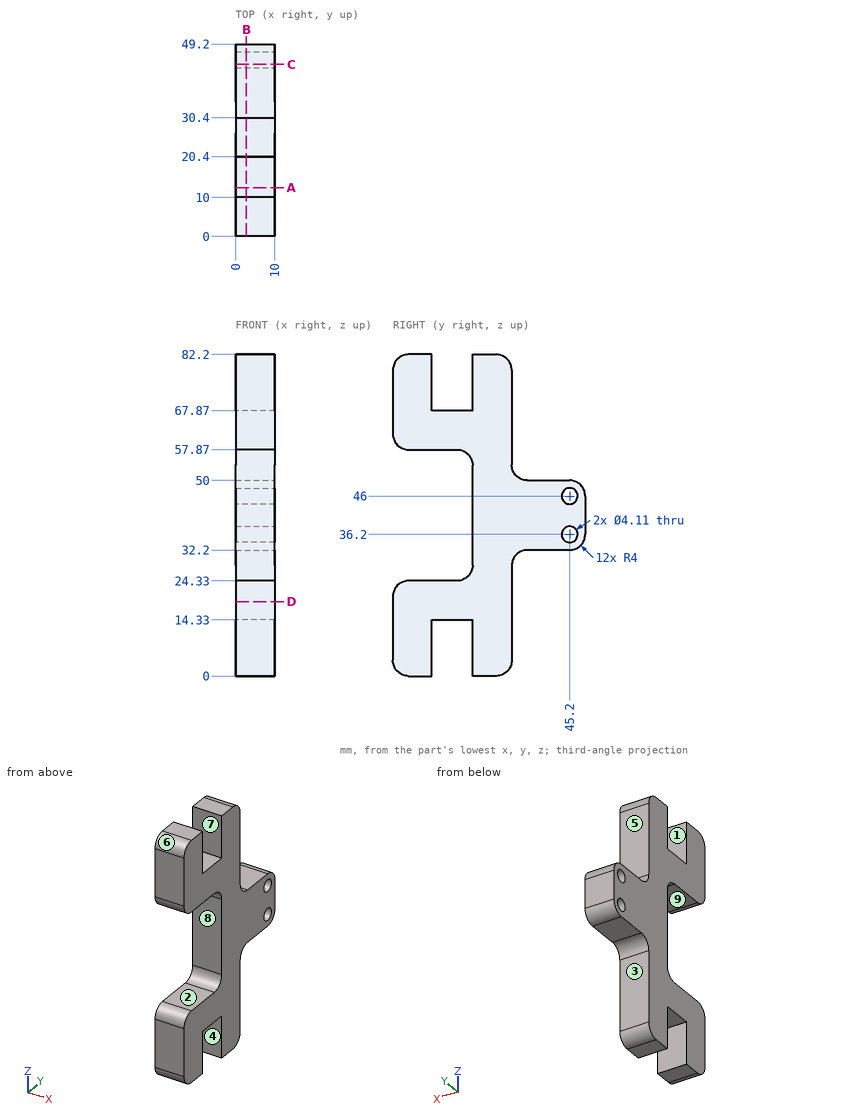
Drawing for the job (mm, zero at the part's lowest x, y, z). A direction names the side the tool comes from. Round coordinates to 2 decimals unless told otherwise and drop trailing zeros. Loops run counter-clockwise (first coordinate to the right, second up) from the corner with the lowest first, then second, coordinate; pieces in that order, holes last. Notation, with made-up numbers: M 45,0.25 L 65,0.25 A11 ccw 65,9.25 Z; hole C -29,63 d10. An arc over 180 degrees is marked long. Use a Markdown table: item, result. Add a question column.
(1) Flat gauge pins, fed straight in: pin 1 (5 mm diameter, centred on x = 4, y = 39, fed in from +Z); pin 2 (6 mm diameter, centred on y = 19.5, z = 52, fed in from -X); pin 3 (6 mm diameter, centred on x = 3.5, y = 16.5, fed in from -Z); pin 4 (3 mm diameter, centred on x = 6, z = 71.5, fed in from +Y). Where does each tip first touch, or does it go through?
(2) Drill centre lines: line 1 (Y direction, x = 3, z = 13); line 2 (Y direction, x = 7.25, z = 46) (3 decimals); line 3 (Z direction, x = 2.25, y = 13.5). Where is each one in solid material? Low to high.
(3) Cut at A-A (y = 12.5). Give the cut face in (x, z), and give its area (3 significant figures).
(4) Cut at D-D (z = 19). Give the cut face in (x, y), and give its area (3 significant figures).
(5) Pull direction Z, two halves, no side cores. Call the marked faces 6, 7, 8 and 9: +Z half, -Z half, draft (parallel to the pull), parting line (faces both ways), or undercut.
(6) Which spindle directions (+Z, -Z, +X, -X, +Y, -Y) get a long thin tool onto all of the face, cutting with end or side? Do the marked faces 1, 2, 3, 4 and 5. Say none if no direction does.
(7) Cut at B-B (x = 2.75). State how many separate pieces and enclosed holes the cut face has, and give its area (3 significant figures).
(8) Cut at C-C (y = 44). Give the cut face in (x, z).
Geometry says:
| question | item | result |
|---|---|---|
| 1 | pin 1 | stops at z = 50 |
| 1 | pin 2 | stops at x = 0 |
| 1 | pin 3 | stops at z = 14.33 |
| 1 | pin 4 | stops at y = 30.4 |
| 2 | line 1 | y = 0 to 10, 20.4 to 30.4 |
| 2 | line 2 | y = 20.4 to 43.145, 47.255 to 49.2 |
| 2 | line 3 | z = 14.33 to 24.33, 57.87 to 67.87 |
| 3 | outline | M 0,14.33 L 10,14.33 L 10,24.33 L 0,24.33 Z; M 0,57.87 L 10,57.87 L 10,67.87 L 0,67.87 Z |
| 3 | area | 200 mm² |
| 4 | outline | M 0,0 L 10,0 L 10,30.4 L 0,30.4 Z |
| 4 | area | 304 mm² |
| 5 | face 6 | +Z half |
| 5 | face 7 | draft |
| 5 | face 8 | undercut |
| 5 | face 9 | undercut |
| 6 | face 1 | +Z, +X, -X |
| 6 | face 2 | +X, -X, -Y |
| 6 | face 3 | -Z, +X, -X, +Y |
| 6 | face 4 | -Z, +X, -X |
| 6 | face 5 | +Z, +X, -X, +Y |
| 7 | separate pieces | 1 |
| 7 | enclosed holes | 2 |
| 7 | area | 1,810 mm² |
| 8 | outline | M 0,32.2 L 10,32.2 L 10,34.53 L 0,34.53 Z; M 0,37.87 L 10,37.87 L 10,44.33 L 0,44.33 Z; M 0,47.67 L 10,47.67 L 10,50 L 0,50 Z |
